Source: three-view drawing plus pictorial views. Frame: mm from the lowest corner of the part. A direction names the side the tool comes from. Coordinates: 2 decimals unless noted, no trailing zeros. Write each loop counter-clockwise with the first axis right and the second up, starting at its lowest first coordinate (ties: lowest second). Pieces come first, ordered by that corner, then holes. Notation, with made-up numbers: (64, -31) - (105, -31) arc R11 ccw to (105, -27) - close; hole circle Ø7 at (-18, -28.75). An arc over 180 degrees is marked (long way). One line per item, written item: value.
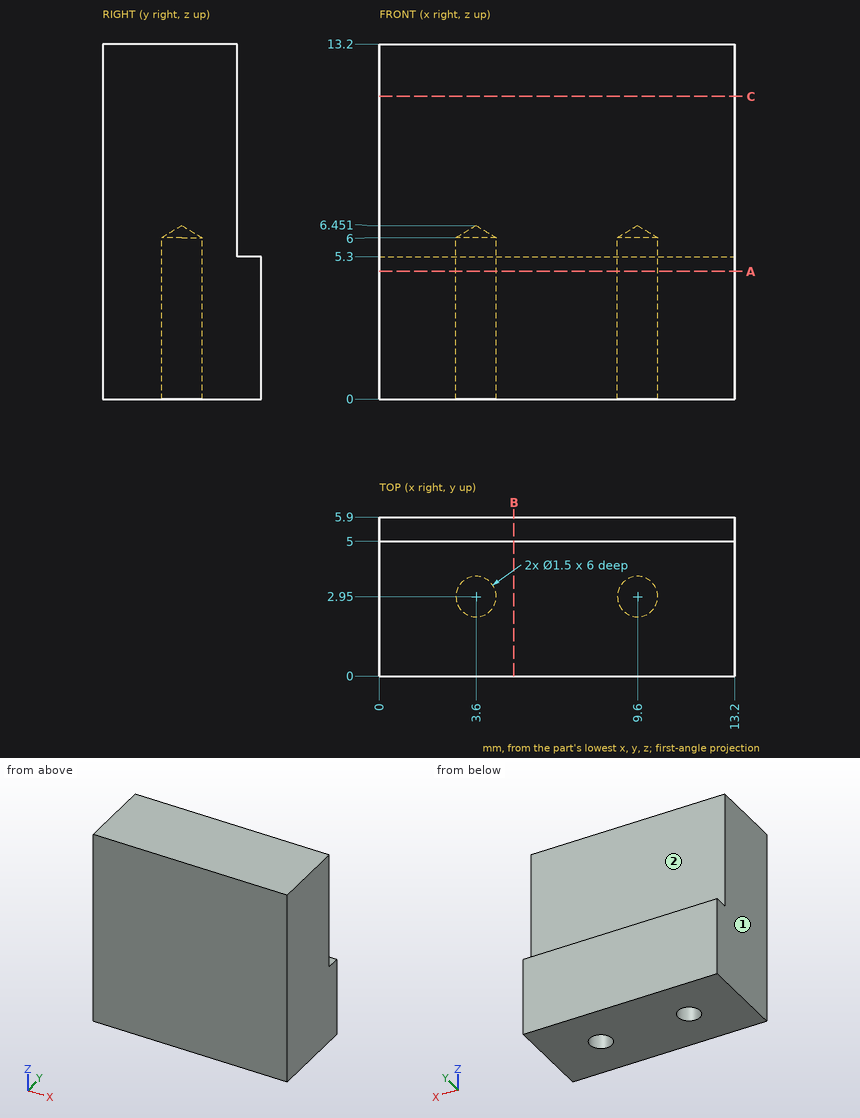
1) Section query A-A on z = 4.75. Output: boundary loops of the cut face in (x, y).
Values found:
outline: (0, 0) - (13.2, 0) - (13.2, 5.9) - (0, 5.9) - close; hole circle Ø1.5 at (3.6, 2.95); hole circle Ø1.5 at (9.6, 2.95)
2) Reachability of the marked faces 1 and 2 from +Z, -Z, +X, -X, +Y, -Y: full face, straight path, thin tool, end or side. Return the list, or none.
Values found:
face 1: +Z, -Z, -X, +Y, -Y
face 2: +Z, +X, -X, +Y
3) Section query B-B on x = 5. Output: boundary loops of the cut face in (y, z).
Values found:
outline: (0, 0) - (5.9, 0) - (5.9, 5.3) - (5, 5.3) - (5, 13.2) - (0, 13.2) - close
4) Material intervals for line 1 (X direction, y = 2.95, z = 1.6); line 2 (Y direction, x = 3.6, z = 4.45); line 3 (Y direction, x = 9.5, z = 9.5), sorted ascending.
Values found:
line 1: 0 to 2.85, 4.35 to 8.85, 10.35 to 13.2
line 2: 0 to 2.2, 3.7 to 5.9
line 3: 0 to 5
5) Section query C-C on z = 11.25. Output: boundary loops of the cut face in (x, y).
Values found:
outline: (0, 0) - (13.2, 0) - (13.2, 5) - (0, 5) - close
6) Contact query for flat-ended pins moving along their axis: P1, Ø0.7, axis at x = 6, y = 5.5, coming from the +Z side; P2, Ø1.5, axis at x = 9.5, z = 10.5, coming from the +Y side. Output: stop coordinate, or through.
Values found:
P1: z = 5.3
P2: y = 5
